```python
from build123d import *

# Parameters (mm, degrees)
BOSS_EXTRUDE1_DEPTH = 1.5
BOSS_EXTRUDE2_DEPTH = 3
SKETCH6_R           = 18
CUT_EXTRUDE1_DEPTH  = 119.782364011


with BuildPart() as part:
    # Sketch3 → Boss-Extrude1 (new body)
    with BuildSketch(Plane.XY):
        with BuildLine():
            Line((-20, 0), (-20, -97))
            ThreePointArc((-20, -97), (0, -117), (20, -97))
            Line((20, -97), (20, 0))
            ThreePointArc((20, 0), (0, 20), (-20, 0))
        make_face()
    extrude(amount=BOSS_EXTRUDE1_DEPTH)

    # Sketch5 → Boss-Extrude2 (add)
    with BuildSketch(Plane.XY.offset(1.5)):
        with BuildLine():
            Line((-19, 0), (-19, -97))
            ThreePointArc((-19, -97), (0, -116), (19, -97))
            Line((19, -97), (19, 0))
            ThreePointArc((19, 0), (0, 19), (-19, 0))
        make_face()
        with BuildLine():
            Line((-18, 0), (-18, -97))
            ThreePointArc((-18, -97), (0, -115), (18, -97))
            Line((18, -97), (18, 0))
            ThreePointArc((18, 0), (0, 18), (-18, 0))
        make_face(mode=Mode.SUBTRACT)
    extrude(amount=BOSS_EXTRUDE2_DEPTH)

    # Sketch6 → Cut-Extrude1 (cut, through all)
    with BuildSketch(Plane(origin=(0, 0, 0), x_dir=(-1, 0, 0), z_dir=(0, 0, -1))):
        with Locations((0, -97)):
            Circle(SKETCH6_R)
    extrude(amount=-CUT_EXTRUDE1_DEPTH, mode=Mode.SUBTRACT)


solid = part.part
```
Source: CAD feature listing. Evaluate the final solid. Frame: model axes, mm. A direction names the side the tool comes from. Give positions to 0.01 mm unless a question says otherwise; leave off trailing zeros. Loops run counter-clockwise (first coordinate to the right, second up) from the corner with the lowest first, then second, coordinate; pieces in that order, holes last. Notation, with made-up numbers: M -9.75,46 L -3.75,46 A27 ccw -3.75,64 Z; hole C 63.5,59.25 d4. An arc over 180 degrees is marked long. Put each result on its own line as item: value.
Q1. Section B-B (z = 2.5). Return the cut outline in (x, y).
Response values:
outline: M -19,-97 A19 ccw 19,-97 L 19,0 A19 ccw -19,0 Z; hole M -18,-97 A18 ccw 18,-97 L 18,0 A18 ccw -18,0 Z
Q2. Pin query (flat end, axial travel): P1, Ø5, axis at x = -9.5, y = -5, coming from the +Z side; P2, Ø0.9, axis at y = -70, z = 2.5, coming from the +X side; P3, Ø0.9, axis at y = -46.5, z = 3, coming from the -X side; P4, Ø21.5, axis at x = 0, y = -97, coming from the +Z side. Return the tip coordinate at first contact, or that it passes through.
Response values:
P1: stops at z = 1.5
P2: stops at x = 19
P3: stops at x = -19
P4: passes through
Q3. Line query: probe 1 along Y at (x, z) = (0, 2.25); probe 2 along Y at (x, z) = (-0.5, 0.9); probe 3 along X at (y, z) = (-58.5, 2.1). Output: solid intervals per line, ascending. Write a range as [from, to].
Response values:
probe 1: y = [-116, -115], [18, 19]
probe 2: y = [-116.99, -114.99], [-79.01, 19.99]
probe 3: x = [-19, -18], [18, 19]
Q4. Mould query, pull axis Y, two halves, no side actions, for faces 4 (the flat face through (-18, -48, 3)), 5 (the cylindrical face through (0, 20, 1)), 6 (the cylindrical face through (0, -117, 1)), 7 (the flat face through (19.2, -48.2, 1.5)). Classes: released by +Y, released by -Y, zero draft, split by the parting line, or undercut.
Response values:
face 4: undercut
face 5: released by +Y
face 6: released by -Y
face 7: zero draft
Q5. Reachability of faces 1 (the flat face through (-19, -48, 3)), 2 (the cylindrical face through (0, -116, 3)), 3 (the flat face through (18, -49, 3)) from +Z, -Z, +X, -X, +Y, -Y: full face, straight path, thin tool, end or side. Return the list, or none.
Response values:
face 1: +Z, -X, +Y, -Y
face 2: +Z, -Y
face 3: +Z
Q6. Section D-D (y = -57). Return the cut outline in (x, z).
Response values:
outline: M -20,0 L 20,0 L 20,1.5 L 19,1.5 L 19,4.5 L 18,4.5 L 18,1.5 L -18,1.5 L -18,4.5 L -19,4.5 L -19,1.5 L -20,1.5 Z
Q7. Section C-C (y = -89). Return the cut outline in (x, z).
Response values:
outline: M -20,0 L -16.12,0 L -16.12,1.5 L -18,1.5 L -18,4.5 L -19,4.5 L -19,1.5 L -20,1.5 Z; M 16.12,0 L 20,0 L 20,1.5 L 19,1.5 L 19,4.5 L 18,4.5 L 18,1.5 L 16.12,1.5 Z
Q8. Section A-A (x = 0). Return the cut outline in (y, z), and give its area (4 significant figures).
Response values:
outline: M -117,0 L -115,0 L -115,4.5 L -116,4.5 L -116,1.5 L -117,1.5 Z; M -79,0 L 20,0 L 20,1.5 L 19,1.5 L 19,4.5 L 18,4.5 L 18,1.5 L -79,1.5 Z
area: 157.5 mm²
